The model under review builds one solid part; all positions refer to its coordinate system, in mm. A direction names the side the tool comes from. Round coordinates to 2 decimals unless told otherwise and drop trailing zeros. Loops run counter-clockwise (first coordinate to the right, second up) from the corner with the lowest first, then second, coordinate; pieces in that order, holes last. Notation, with made-up numbers: M -34.75,12 L -5.75,12 A23 ccw -5.75,33 Z; hole C -1,-16.75 d4. An arc over 180 degrees is marked long. Return JSON: item names as keys, results as strings. Group by question number.
Q1. Consider section D-D (y = 13). State the section outline as (x, z) points, and give its area (3 significant figures).
Q2. Consider section C-C (x = 5.5). State the section outline as (y, z) points, and give its area (3 significant figures).
Q3. For faces 1 (the face through (20, 28, 5)), 2 (the face through (20, 0, 65)), list the 3-axis set-ups (+Z, -Z, +X, -X, +Y, -Y) from which the entire face can be reached by the end or side of a thin tool; tool diameter is ignored.
Q4. To check wall thickness, follow line 1 along X through (y, z) = (2.15, 101); line 2 along Y through (x, z) = (10, 3); line 3 along Y through (x, z) = (30, 1.9). State the ranges of each line that lie inside material, in increasing order.
Q5. Draft analysis for pull direction X (two halves, no side actions). For faces 3 (the face through (20.224, 1.141, 1.203)), 4 (the face through (38.797, 4.507, 129.859)), 5 (the face through (9.67, 2.46, 123.48)), state which applies: pulls with the +X half, pulls with the -X half, needs draft (parallel to the pull), parting line crosses it, or undercut.
Q6. Clearance check with flat-ended pins moving along their axes: pin 1 Ø6.5 at (x, z) = (10, 101) entering from +Y; pin 2 Ø6 at (x, y) = (30, 41) entering from +Z; pin 3 Ø10 at (x, z) = (14.5, 26) entering from -Y; pin 4 Ø4.5 at (x, y) = (30, 21) entering from -Z. State where each tip first meets the part, or that it passes through.
Q7. Consider section A-A (z = 121). State the section outline as (x, y) points, and give its area (3 significant figures).
Autodesk Fusion 360 part; units mm, degrees
sketch "Sketch1" plane through (0, 0, 0) normal (0, 0, 1) x (1, 0, 0)
  line L0 (0, 0) -> (40, 0)
  line L1 (40, 0) -> (40, 51)
  line L2 (40, 51) -> (0, 51)
  line L3 (0, 51) -> (0, 0)
  dimension "d1" = 40
  dimension "d2" = 51
extrude "Extrude1" add sketch "Sketch1" along normal blind 5
sketch "Sketch2" plane through (0, 0, 5) normal (0, 0, 1) x (-1, 0, 0)
  line L0 (0, -51) -> (0, 0)
  line L1 (0, 0) -> (-40, 0)
  line L2 (-40, 0) -> (-40, -51)
  line L3 (-40, -51) -> (0, -51)
  line L4 (0, 0) -> (-40, 0)
  line L5 (-40, 0) -> (-40, -5)
  line L6 (-40, -5) -> (0, -5)
  line L7 (0, -5) -> (0, 0)
  dimension "d5" = 40
  dimension "d6" = 5
extrude "Extrude2" add sketch "Sketch2" along normal blind 126 contours L0 L1 L2 L4 L5 L6 L7
sketch "Sketch3" plane through (0, 0, 0) normal (0, -1, 0) x (1, 0, 0)
  line L0 (0, 0) -> (40, 0)
  line L1 (40, 0) -> (40, 131)
  line L2 (40, 131) -> (0, 131)
  line L3 (0, 131) -> (0, 0)
  line L4 (0, 131) -> (10, 131)
  line L5 (10, 131) -> (10, 121)
  line L6 (10, 121) -> (0, 121)
  line L7 (0, 121) -> (0, 131)
  circle A0 centre (10, 121) radius 2.5
  line L8 (10, 121) -> (30, 121)
  line L9 (30, 121) -> (30, 101)
  line L10 (30, 101) -> (10, 101)
  line L11 (10, 101) -> (10, 121)
  circle A1 centre (30, 121) radius 2.5
  circle A2 centre (10, 101) radius 2.5
  circle A3 centre (30, 101) radius 2.5
  dimension "d9" = 10
  dimension "d10" = 10
  dimension "d11" = 5
  dimension "d12" = 20
  dimension "d13" = 20
  dimension "d14" = 5
  dimension "d15" = 5
  dimension "d16" = 5
extrude "Extrude3" cut sketch "Sketch3" against normal blind 5 contours L5 L6 A0 | L6 A0 L11 | L5 A0 L8 | A0 L8 L11 | L10 L11 A2 | L10 L11 A2 | L8 L9 A1 | L8 L9 A1 | L9 L10 A3 | L9 L10 A3
sketch "Sketch4" plane through (0, 0, 5) normal (0, 0, 1) x (-1, 0, 0)
  line L0 (0, -5) -> (-40, -5)
  line L1 (-40, -5) -> (-40, -51)
  line L2 (-40, -51) -> (0, -51)
  line L3 (0, -51) -> (0, -5)
  line L4 (0, -51) -> (-10, -51)
  line L5 (-10, -51) -> (-10, -41)
  line L6 (-10, -41) -> (0, -41)
  line L7 (0, -41) -> (0, -51)
  line L8 (-10, -41) -> (-30, -41)
  line L9 (-30, -41) -> (-30, -21)
  line L10 (-30, -21) -> (-10, -21)
  line L11 (-10, -21) -> (-10, -41)
  circle A0 centre (-10, -41) radius 2.5
  circle A1 centre (-30, -41) radius 2.5
  circle A2 centre (-10, -21) radius 2.5
  circle A3 centre (-30, -21) radius 2.5
  dimension "d19" = 10
  dimension "d20" = 10
  dimension "d21" = 20
  dimension "d22" = 20
  dimension "d23" = 5
  dimension "d24" = 5
  dimension "d25" = 5
  dimension "d26" = 5
extrude "Extrude4" cut sketch "Sketch4" against normal blind 5 contours L5 L6 A0 | L6 L11 A0 | L5 L8 A0 | L8 L11 A0 | L10 L11 A2 | L10 L11 A2 | L8 L9 A1 | L8 L9 A1 | L9 L10 A3 | L9 L10 A3
fillet "Fillet1" radius 4 11 edges at (40, 25.5, 0) (20, 0, 0) (20, 51, 0) (40, 51, 2.5) (0, 51, 2.5) (0, 25.5, 0) (40, 0, 65.5) (40, 2.5, 131) (0, 0, 65.5) (0, 2.5, 131) (20, 0, 131)
Values:
{
 "1": {"outline": "M 0,4 A4 ccw 4,0 L 36,0 A4 ccw 40,4 L 40,5 L 0,5 Z", "area": "193 mm2"},
 "2": {"outline": "M 0,4 A4 ccw 4,0 L 47,0 A4 ccw 51,4 L 51,5 L 5,5 L 5,131 L 4,131 A4 ccw 0,127 Z", "area": "875 mm2"},
 "3": {"face 1": "+Z, +X, -X, +Y", "face 2": "+Z, -Z, +X, -X, -Y"},
 "4": {"line 1": "x = 0.45 to 7.5, 12.5 to 27.5, 32.5 to 39.55", "line 2": "y = 0.13 to 18.5, 23.5 to 38.5, 43.5 to 50.87", "line 3": "y = 0.6 to 18.5, 23.5 to 38.5, 43.5 to 50.4"},
 "5": {"face 3": "needs draft", "face 4": "pulls with the +X half", "face 5": "undercut"},
 "6": {"pin 1": "stops at y = 5", "pin 2": "stops at z = 5", "pin 3": "stops at y = 0", "pin 4": "passes through"},
 "7": {"outline": "M 0,4 A4 ccw 4,0 L 7.5,0 L 7.5,5 L 0,5 Z; M 12.5,0 L 27.5,0 L 27.5,5 L 12.5,5 Z; M 32.5,0 L 36,0 A4 ccw 40,4 L 40,5 L 32.5,5 Z", "area": "143 mm2"}
}
